Model file for the job. Use its own axes, mm. Face numbers are marked on the shaded views. Coordinates: 2 decimals unless noted, no trailing zeros. Order: outer loops, then holes, each group sorted by start corner. A loop starts at its lowest first (then second) coordinate and runs counter-clockwise, first axis right, second up.
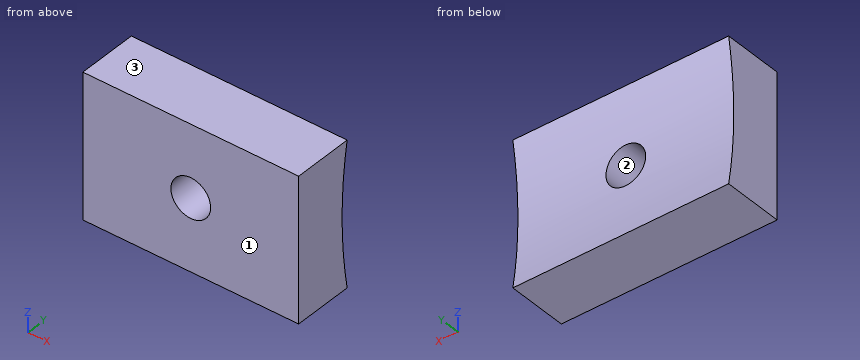
from build123d import *

# Parameters (mm, degrees)
SKETCH1_W                       = 19.05
SKETCH1_H                       = 12.7
EXTRUDE1_DEPTH                  = 41.275
SKETCH2_R                       = 36.5125
CUT_EXTRUDE1_DEPTH              = 41.275
F_6_32_TAPPED_HOLE1_D           = 2.7051
F_6_32_TAPPED_HOLE1_DEPTH       = 9.398
F_6_32_TAPPED_HOLE1_CBORE_D     = 3.5052
F_6_32_TAPPED_HOLE1_CBORE_DEPTH = 7.112
F_6_32_TAPPED_HOLE1_TIP         = 0.81269403


with BuildPart() as part:
    # Sketch1 → Extrude1 (new body)
    with BuildSketch(Plane(origin=(0, 0, 0), x_dir=(1, 0, 0), z_dir=(0, 1, 0))):
        Rectangle(SKETCH1_W, SKETCH1_H)
    extrude(amount=EXTRUDE1_DEPTH)

    # Sketch2 → Cut-Extrude1 (cut)
    with BuildSketch(Plane.ZY.offset(9.525)):
        with Locations((0, 41.275)):
            Circle(SKETCH2_R)
    extrude(amount=-CUT_EXTRUDE1_DEPTH, mode=Mode.SUBTRACT)

    # #6-32 Tapped Hole1
    with Locations(Plane(origin=(0, 0, 0), x_dir=(0, 0, -1), z_dir=(0, -1, 0))):
        with Locations((0, 0)):
            CounterBoreHole(F_6_32_TAPPED_HOLE1_D / 2, F_6_32_TAPPED_HOLE1_CBORE_D / 2, F_6_32_TAPPED_HOLE1_CBORE_DEPTH, depth=F_6_32_TAPPED_HOLE1_DEPTH)
            with Locations((0, 0, -(F_6_32_TAPPED_HOLE1_DEPTH + F_6_32_TAPPED_HOLE1_TIP / 2))):  # 118° drill point
                Cone(0, F_6_32_TAPPED_HOLE1_D / 2, F_6_32_TAPPED_HOLE1_TIP, mode=Mode.SUBTRACT)


solid = part.part
Q1. Probe line 1 (Z direction, x = 0, y = 2.95); line 2 (X direction, y = 3.65, z = 0) (3 decimals); line 3 (Y direction, x = 0.75, z = 1.75). List the from-to ranges inside material, lowest first.
Established:
line 1: z = -6.35 to -1.75, 1.75 to 6.35
line 2: x = -9.525 to -1.753, 1.753 to 9.525
line 3: y = 0 to 4.8
Q2. Mould opens along Z. For the marked faces 1, 2 and 3 say: pulls with the +Z half, pulls with the -Z half, needs draft (parallel to the pull), parting line crosses it, or undercut.
Established:
face 1: needs draft
face 2: undercut
face 3: pulls with the +Z half
Q3. Drop a flat-ended pin along its axis: P1, Ø1.5, axis at x = -2, z = 2.5, coming from the -Y side. Give the stop position or say it passes through.
Established:
P1: stops at y = 0
Q4. Cut at A-A, the plane z = 0. List the corners of the cut face in (x, y) (1 decimal).
Established:
outline: (-9.5, 0) - (-1.8, 0) - (-1.8, 4.8) - (-9.5, 4.8) - close; (1.8, 0) - (9.5, 0) - (9.5, 4.8) - (1.8, 4.8) - close
Q5. Cut at C-C, the plane y = 2.5. List the corners of the cut face in (x, z) (3 decimals).
Established:
outline: (-9.525, -6.35) - (9.525, -6.35) - (9.525, 6.35) - (-9.525, 6.35) - close; hole circle Ø3.505 at (0, 0)
